from build123d import *

# Parameters (mm, degrees)
SKETCH1_R           = 3.175
BOSS_EXTRUDE1_DEPTH = 3.175
FILLET1_R           = 7.62
FILLET2_R           = 2.54


with BuildPart() as part:
    # Sketch1 → Boss-Extrude1 (new body)
    with BuildSketch(Plane(origin=(0, 0, 0), x_dir=(1, 0, 0), z_dir=(0, 1, 0))):
        Polygon((-12.7, -6.35), (-12.7, 6.35), (12.7, 6.35), (12.7, -6.35), (0, -15.875), align=None)
        with Locations(Location((-0.266746272, -6.35, 0), (0, 0, 270))):
            Circle(SKETCH1_R, mode=Mode.SUBTRACT)
    extrude(amount=BOSS_EXTRUDE1_DEPTH)

    # Fillet1
    fillet1_edges = [part.edges().sort_by_distance(p)[0] for p in [
        (0, 1.5875, 15.875),
    ]]
    fillet(fillet1_edges, radius=FILLET1_R)

    # Fillet2
    fillet2_edges = [part.edges().sort_by_distance(p)[0] for p in [
        (12.7, 1.5875, 6.35),
        (-12.7, 1.5875, 6.35),
    ]]
    fillet(fillet2_edges, radius=FILLET2_R)


solid = part.part
Geometry check sheet. Reference: the model listing, model coordinates, mm. Round coordinates to 2 decimals unless told otherwise and drop trailing zeros. Write each loop counter-clockwise with the first axis right and the second up, starting at its lowest first coordinate (ties: lowest second). Pieces come first, ordered by that corner, then holes.
Item 1: Go/stop test with flat-tipped pins: pin 1 Ø10 at (x, z) = (-9.5, -2) entering from -Y; pin 2 Ø1.5 at (y, z) = (1, 11) entering from -X. Record where each tip stops, or that it passes through.
Determined:
pin 1: stops at y = 0
pin 2: stops at x = -7.5
Item 2: Section check A-A (x = 0.5). Record the boundary of the cut face in (y, z) (3 decimals), plus the area to 3 significant figures.
Determined:
outline: (0, -6.35) - (3.175, -6.35) - (3.175, 3.269) - (0, 3.269) - close; (0, 9.431) - (3.175, 9.431) - (3.175, 13.954) - (0, 13.954) - close
area: 44.9 mm2
Item 3: Section check C-C (y = 1.85). Record the boundary of the cut face in (x, z) (3 decimals).
Determined:
outline: (-12.7, -6.35) - (12.7, -6.35) - (12.7, 5.08) arc R2.54 ccw to (11.684, 7.112) - (4.572, 12.446) arc R7.62 ccw to (-4.572, 12.446) - (-11.684, 7.112) arc R2.54 ccw to (-12.7, 5.08) - close; hole circle Ø6.35 at (-0.267, 6.35)
Item 4: Material ranges on line 1 along Z through (x, y) = (1.25, 2); line 2 along X through (y, z) = (0.75, 6.35); line 3 along Z through (x, y) = (-2.5, 1.5), recorded low to high.
Determined:
line 1: z = -6.35 to 3.56, 9.14 to 13.87
line 2: x = -12.36 to -3.44, 2.91 to 12.36
line 3: z = -6.35 to 4.09, 8.61 to 13.55
Item 5: Section check D-D (x = -9.5). Record the boundary of the cut face in (y, z) (3 decimals), plus the area to 3 significant figures.
Determined:
outline: (0, -6.35) - (3.175, -6.35) - (3.175, 8.75) - (0, 8.75) - close
area: 47.9 mm2
Item 6: Mould release check, pull along Z, two halves, no side actions. Record for faces 1 (the face through (0, 2, -6.35)), 2 (the face through (-0.127, 1.565, 3.178)), 3 (the face through (12.424, 1.61, 6.231)): +Z half, -Z half, draft (parallel to the pull), parting line (faces both ways), or undercut.
Determined:
face 1: -Z half
face 2: undercut
face 3: +Z half
Item 7: Section check B-B (z = 6.35). Record the boundary of the cut face in (x, y) (3 decimals).
Determined:
outline: (-12.36, 0) - (-3.442, 0) - (-3.442, 3.175) - (-12.36, 3.175) - close; (2.908, 0) - (12.36, 0) - (12.36, 3.175) - (2.908, 3.175) - close
